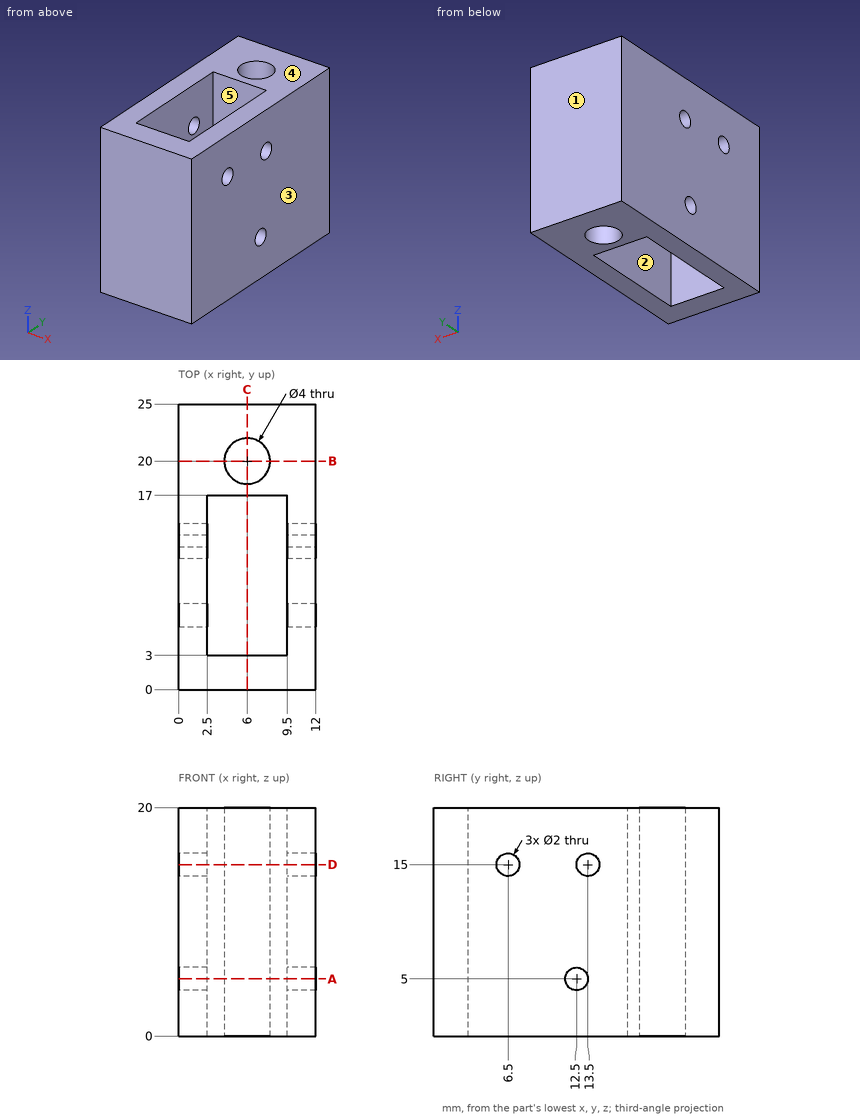
Could you check a few things on this drawing? It's one solid part, dimensions in mm from its lowest x, y, z. A direction names the side the tool comes from. Coordinates: 2 decimals unless noted, no trailing zeros. Loops run counter-clockwise (first coordinate to the right, second up) from the corner with the lowest first, then second, coordinate; pieces in that order, holes last. Notation, with made-up numbers: (11, 3.25) - (62, 3.25) arc R20 ccw to (62, 7.25) - close; hole circle Ø3 at (11.25, 74.25). An arc over 180 degrees is marked (long way). Return JSON: item names as keys, results as strings. Group by question number.
Item 1: If we section it at C-C on x = 6: Write out the boundary of the cut face in (y, z).
Item 2: On a 3-axis mill with a long thin cutter (end or side, diameter ignored), from which of +Z, -Z, +X, -X, +Y, -Y can I reach the whole of each face in a straight line? I mean the marked faces 1 and 2. Say none if no direction works.
Item 3: If we section it at A-A on z = 5: Write out the boundary of the cut face in (x, y).
Item 4: I need wall thicknesses on line 1 (Y direction, x = 6, z = 4.75); line 2 (X direction, y = 8.25, z = 4); line 3 (Z direction, x = 10.3, y = 6.5). Which ranges of each line are inside material? Lowest first, please. Write a range as from..to.
Item 5: Will these pins go through, and if not, where does the flat tip stop? P1, Ø4, axis at x = 6, y = 10, coming from the -Z side; P2, Ø3.5, axis at x = 6, z = 11, coming from the -Y side.
Item 6: If we section it at D-D on z = 15: Write out the boundary of the cut face in (x, y), and give its area (3 significant figures).
Item 7: We'd pull the mould along X, two halves only. Please class the marked faces 3, 4 and 5: +X half, -X half, draft (parallel to the pull), parting line (faces both ways), or undercut.
Item 8: If we section it at B-B on y = 20: Write out the boundary of the cut face in (x, z).
Calculated:
{
 "1": {"outline": "(0, 0) - (3, 0) - (3, 20) - (0, 20) - close; (17, 0) - (18, 0) - (18, 20) - (17, 20) - close; (22, 0) - (25, 0) - (25, 20) - (22, 20) - close"},
 "2": {"face 1": "+Z, -Z, +X, -X, +Y", "face 2": "+Z, -Z"},
 "3": {"outline": "(0, 0) - (12, 0) - (12, 11.5) - (9.5, 11.5) - (9.5, 3) - (2.5, 3) - (2.5, 11.5) - (0, 11.5) - close; (0, 13.5) - (2.5, 13.5) - (2.5, 17) - (9.5, 17) - (9.5, 13.5) - (12, 13.5) - (12, 25) - (0, 25) - close; hole circle Ø4 at (6, 20)"},
 "4": {"line 1": "y = 0..3, 17..18, 22..25", "line 2": "x = 0..2.5, 9.5..12", "line 3": "z = 0..14, 16..20"},
 "5": {"P1": "passes through", "P2": "stops at y = 0"},
 "6": {"outline": "(0, 0) - (12, 0) - (12, 5.5) - (9.5, 5.5) - (9.5, 3) - (2.5, 3) - (2.5, 5.5) - (0, 5.5) - close; (0, 7.5) - (2.5, 7.5) - (2.5, 12.5) - (0, 12.5) - close; (0, 14.5) - (2.5, 14.5) - (2.5, 17) - (9.5, 17) - (9.5, 14.5) - (12, 14.5) - (12, 25) - (0, 25) - close; (9.5, 7.5) - (12, 7.5) - (12, 12.5) - (9.5, 12.5) - close; hole circle Ø4 at (6, 20)", "area": "169 mm^2"},
 "7": {"face 3": "+X half", "face 4": "draft", "face 5": "undercut"},
 "8": {"outline": "(0, 0) - (4, 0) - (4, 20) - (0, 20) - close; (8, 0) - (12, 0) - (12, 20) - (8, 20) - close"}
}
